Here's how the part is built. I have some questions about the finished solid (model axes, mm). A direction names the side the tool comes from. Round coordinates to 2 decimals unless told otherwise and drop trailing zeros. Write each loop counter-clockwise with the first axis right and the second up, starting at its lowest first coordinate (ties: lowest second). Pieces come first, ordered by that corner, then holes. Notation, with made-up numbers: (-22.5, 75) -> (-2.5, 75) arc R22 cw to (-2.5, 96) -> close; hole circle Ø3 at (-31.75, 78). An arc over 180 degrees is marked (long way). Put each result on its own line as item: value. Start each with the question number.
1) If I drill on line 1 along X through (y, z) = (29.5, -1.75); line 2 along Y through (x, z) = (-3.5, -2.25); line 3 along X through (y, z) = (-0.5, 1.25), over which ranges is the centre line in solid material (lowest first)? Write a range as [from, to].
2) Will these pins go through, and if not, where does the flat tip stop? P1, Ø2.5, axis at x = -3, y = 30, coming from the -Z side; P2, Ø6, axis at x = 14.5, z = -8, coming from the -Y side; P3, Ø18.5, axis at x = 7.5, y = 7.5, coming from the -Z side; P4, Ø12, axis at y = 17.5, z = -7.5, coming from the +X side.
3) I want a section at A-A, the plane y = 26.5. List the corners of the cut face in (x, z) for me.
4) Which directions (+Z, -Z, +X, -X, +Y, -Y) give clear straight access to the entire face, cutting with the end or side of a thin tool? Please do faces 1 (the flat face through (0, 29, 8)), 2 (the flat face through (0, 0, 0)), 3 (the flat face through (0, 7, -7.5)), 4 (the flat face through (0, 7, 7.5)), 5 (the flat face through (10.5, 28, 0)).
5) We'd pull the mould along X, two halves only. Please class faces 6 (the flat face through (-7.5, 29, -2)), 7 (the flat face through (27, -4, 0)), 8 (the flat face through (-10.5, 28, 0)): released by +X, released by -X, zero draft, split by the parting line, or undercut.
6) I want a section at B-B, the plane y = 9. List the corners of the cut face in (x, z) for me.
from build123d import *

# Parameters (mm, degrees)
SKETCH1_W           = 60
SKETCH1_H           = 15
BOSS_EXTRUDE1_DEPTH = 13
SKETCH4_W           = 5
SKETCH4_H           = 15
BOSS_EXTRUDE2_DEPTH = 4
SKETCH5_W           = 21
SKETCH5_H           = 22
BOSS_EXTRUDE3_DEPTH = 3
BOSS_EXTRUDE4_DEPTH = 3


with BuildPart() as part:
    # Sketch1 → Boss-Extrude1 (new body)
    with BuildSketch(Plane(origin=(0, 0, 0), x_dir=(1, 0, 0), z_dir=(0, 1, 0))):
        Rectangle(SKETCH1_W, SKETCH1_H)
    extrude(amount=BOSS_EXTRUDE1_DEPTH)

    # Sketch4 → Boss-Extrude2 (add)
    with BuildSketch(Plane(origin=(0, 0, 0), x_dir=(-1, 0, 0), z_dir=(0, -1, 0))):
        with Locations((27.5, 0)):
            Rectangle(SKETCH4_W, SKETCH4_H)
    boss_extrude2 = extrude(amount=BOSS_EXTRUDE2_DEPTH)

    # Mirror1: Boss-Extrude2 across plane
    add(boss_extrude2.mirror(Plane(origin=(0, 0, 0), x_dir=(0, 0, 1), z_dir=(1, 0, 0))))



with BuildPart() as body_2:
    # Sketch5 → Boss-Extrude3 (new body)
    with BuildSketch(Plane(origin=(0, 28, 0), x_dir=(-1, 0, 0), z_dir=(0, -1, 0))):
        Rectangle(SKETCH5_W, SKETCH5_H)
    extrude(amount=BOSS_EXTRUDE3_DEPTH)


with BuildPart() as part_1:
    add(part.part)

    add(body_2.part)  # loft1 joins it to this body
    # loft from a face of the part (loft1)
    loft([part_1.faces().sort_by_distance((0, 13, 0))[0], part_1.faces().sort_by_distance((0, 25, 0))[0]])

    # Sketch7 → Boss-Extrude4 (add)
    with BuildSketch(Plane(origin=(0, 28, 0), x_dir=(-1, 0, 0), z_dir=(0, -1, 0))):
        Polygon((10.5, 11), (7.5, 11), (7.5, -8), (-7.5, -8), (-7.5, 11), (-10.5, 11), (-10.5, -11), (10.5, -11), align=None)
    extrude(amount=-BOSS_EXTRUDE4_DEPTH)


solid = part_1.part
Findings:
1. line 1: x = [-10.5, -7.5], [7.5, 10.5]
1. line 2: y = [0, 28]
1. line 3: x = [-30, -25], [25, 30]
2. P1: stops at z = 8
2. P2: stops at y = 0
2. P3: stops at z = -8.59
2. P4: stops at x = 30
3. outline: (-10.5, -11) -> (10.5, -11) -> (10.5, 11) -> (-10.5, 11) -> close
4. face 1: -Z, +Y
4. face 2: +Z, -Z, -Y
4. face 3: -Z, +X, -X, -Y
4. face 4: +Z, +X, -X, -Y
4. face 5: +Z, -Z, +X, +Y
5. face 6: undercut
5. face 7: zero draft
5. face 8: released by -X
6. outline: (-30, -7.5) -> (30, -7.5) -> (30, 7.5) -> (-30, 7.5) -> close
